Autodesk Inventor part; units mm, degrees
ref_plane "Work Plane1" through (84.9941, 63.8575, 47) normal (0, 1, 0) x (1, 0, 0)
ref_plane "Work Plane2" through (84.9941, 31.8575, 0) normal (-1, 0, 0) x (0, 0, 1)
ref_plane "YZ Plane" through (0, 0, 0) normal (1, 0, 0) x (0, 1, 0)
sketch "Sketch1" plane through (0, 0, 0) normal (0, 0, 1) x (1, 0, 0)
  line L0 (29.367, 37.7153) -> (29.0801, 37.3058)
  arc A0 (25.6709, 43.8574) -> (29.0801, 37.3058) centre (33.6709, 43.8574) ccw
  line L1 (25.6709, 51.8574) -> (25.6709, 43.8574)
  line L2 (25.6709, 43.8574) -> (25.6709, 51.8574)
  arc A1 (33.6709, 59.8574) -> (25.6709, 51.8574) centre (33.6709, 51.8574) ccw
  line L3 (33.6709, 59.8574) -> (64.6709, 59.8574)
  arc A2 (72.6709, 51.8574) -> (64.6709, 59.8574) centre (64.6709, 51.8574) ccw
  line L4 (72.6709, 43.8574) -> (72.6709, 51.8574)
  line L5 (72.6709, 51.8576) -> (72.6709, 43.8574)
  arc A3 (64.6709, 35.8574) -> (72.6709, 43.8574) centre (64.6709, 43.8574) ccw
  arc A4 (33.6709, 59.8574) -> (25.6709, 51.8574) centre (33.6709, 51.8574) ccw
  arc A5 (25.6709, 43.8574) -> (33.6709, 35.8574) centre (33.6709, 43.8574) ccw
  arc A6 (64.6709, 35.8574) -> (72.6709, 43.8574) centre (64.6709, 43.8574) ccw
  arc A7 (72.6709, 51.8574) -> (64.6709, 59.8574) centre (64.6709, 51.8574) ccw
  line L6 (33.6709, 35.8574) -> (64.6709, 35.8574)
  line L7 (33.6709, 35.8574) -> (50.3633, 35.8574)
  line L8 (50.3633, 59.8574) -> (50.3633, 35.8574)
  line L9 (25.6709, 47.8574) -> (50.3633, 47.8574)
  line L10 (84.9941, 47.8575) -> (84.9941, 63.8575)
  line L11 (84.9941, 63.8575) -> (184.9941, 63.8575)
  line L12 (84.9941, 47.8575) -> (84.9941, 31.8575)
  line L13 (84.9941, 31.8575) -> (184.9941, 31.8575)
  line L14 (184.9941, 31.8575) -> (184.9941, 63.8575)
  line L15 (184.9941, 31.8575) -> (164.9941, 31.8575)
  line L16 (164.9941, 31.8575) -> (164.9941, 21.8575)
  line L17 (164.9941, 21.8575) -> (154.9941, 21.8575)
  line L18 (154.9941, 21.8575) -> (154.9941, 31.8575)
  line L19 (84.9941, 31.8575) -> (104.9941, 31.8575)
  line L20 (104.9941, 31.8575) -> (104.9941, 21.8575)
  line L21 (104.9941, 21.8575) -> (114.9941, 21.8575)
  line L22 (114.9941, 21.8575) -> (114.9941, 31.8575)
  line L23 (184.9941, 63.8575) -> (164.9941, 63.8575)
  line L24 (164.9941, 63.8575) -> (164.9941, 73.8575)
  line L25 (164.9941, 73.8575) -> (154.9941, 73.8575)
  line L26 (154.9941, 73.8575) -> (154.9941, 63.8575)
  line L27 (84.9941, 63.8575) -> (104.9941, 63.8575)
  line L28 (104.9941, 63.8575) -> (104.9941, 73.8575)
  line L29 (104.9941, 73.8575) -> (114.9941, 73.8575)
  line L30 (114.9941, 73.8575) -> (114.9941, 63.8575)
  line L31 (104.9941, 63.8575) -> (109.9941, 63.8575)
  line L32 (104.9941, 31.8575) -> (109.9941, 31.8575)
  line L33 (104.9941, 31.8575) -> (109.9941, 31.8575)
  line L34 (109.9941, 26.8575) -> (109.9941, 31.8575)
  line L35 (154.9941, 63.8575) -> (159.9941, 63.8575)
  line L36 (154.9941, 31.8575) -> (159.9941, 31.8575)
  circle A8 centre (109.9941, 68.8575) radius 1.5875
  circle A9 centre (159.9941, 68.8575) radius 1.5875
  circle A10 centre (109.9941, 26.8575) radius 1.5875
  circle A11 centre (159.9941, 26.8575) radius 1.5875
  point P0 (0, 0)
sketch "Sketch2" plane through (0, 0, 0) normal (0, 0, 1) x (1, 0, 0)
  line L0 (29.367, 37.7153) -> (29.0801, 37.3058)
  arc A0 (25.6709, 43.8574) -> (29.0801, 37.3058) centre (33.6709, 43.8574) ccw
  line L1 (25.6709, 51.8574) -> (25.6709, 43.8574)
  line L2 (25.6709, 43.8574) -> (25.6709, 51.8574)
  arc A1 (33.6709, 59.8574) -> (25.6709, 51.8574) centre (33.6709, 51.8574) ccw
  line L3 (33.6709, 59.8574) -> (64.6709, 59.8574)
  arc A2 (72.6709, 51.8574) -> (64.6709, 59.8574) centre (64.6709, 51.8574) ccw
  line L4 (72.6709, 43.8574) -> (72.6709, 51.8574)
  line L5 (72.6709, 51.8576) -> (72.6709, 43.8574)
  arc A3 (64.6709, 35.8574) -> (72.6709, 43.8574) centre (64.6709, 43.8574) ccw
  arc A4 (33.6709, 59.8574) -> (25.6709, 51.8574) centre (33.6709, 51.8574) ccw
  arc A5 (25.6709, 43.8574) -> (33.6709, 35.8574) centre (33.6709, 43.8574) ccw
  arc A6 (64.6709, 35.8574) -> (72.6709, 43.8574) centre (64.6709, 43.8574) ccw
  arc A7 (72.6709, 51.8574) -> (64.6709, 59.8574) centre (64.6709, 51.8574) ccw
  line L6 (33.6709, 35.8574) -> (64.6709, 35.8574)
  line L7 (33.6709, 35.8574) -> (50.3633, 35.8574)
  line L8 (50.3633, 59.8574) -> (50.3633, 35.8574)
  line L9 (25.6709, 47.8574) -> (50.3633, 47.8574)
  line L10 (84.9941, 47.8575) -> (84.9941, 63.8575)
  line L11 (84.9941, 63.8575) -> (184.9941, 63.8575)
  line L12 (84.9941, 47.8575) -> (84.9941, 31.8575)
  line L13 (84.9941, 31.8575) -> (184.9941, 31.8575)
  line L14 (184.9941, 31.8575) -> (184.9941, 63.8575)
  line L15 (184.9941, 31.8575) -> (164.9941, 31.8575)
  line L16 (164.9941, 31.8575) -> (164.9941, 21.8575)
  line L17 (164.9941, 21.8575) -> (154.9941, 21.8575)
  line L18 (154.9941, 21.8575) -> (154.9941, 31.8575)
  line L19 (84.9941, 31.8575) -> (104.9941, 31.8575)
  line L20 (104.9941, 31.8575) -> (104.9941, 21.8575)
  line L21 (104.9941, 21.8575) -> (114.9941, 21.8575)
  line L22 (114.9941, 21.8575) -> (114.9941, 31.8575)
  line L23 (184.9941, 63.8575) -> (164.9941, 63.8575)
  line L24 (164.9941, 63.8575) -> (164.9941, 73.8575)
  line L25 (164.9941, 73.8575) -> (154.9941, 73.8575)
  line L26 (154.9941, 73.8575) -> (154.9941, 63.8575)
  line L27 (84.9941, 63.8575) -> (104.9941, 63.8575)
  line L28 (104.9941, 63.8575) -> (104.9941, 73.8575)
  line L29 (104.9941, 73.8575) -> (114.9941, 73.8575)
  line L30 (114.9941, 73.8575) -> (114.9941, 63.8575)
  line L31 (104.9941, 63.8575) -> (109.9941, 63.8575)
  line L32 (104.9941, 31.8575) -> (109.9941, 31.8575)
  line L33 (104.9941, 31.8575) -> (109.9941, 31.8575)
  line L34 (109.9941, 26.8575) -> (109.9941, 31.8575)
  line L35 (154.9941, 63.8575) -> (159.9941, 63.8575)
  line L36 (154.9941, 31.8575) -> (159.9941, 31.8575)
  circle A8 centre (109.9941, 68.8575) radius 1.5875
  circle A9 centre (159.9941, 68.8575) radius 1.5875
  circle A10 centre (109.9941, 26.8575) radius 1.5875
  circle A11 centre (159.9941, 26.8575) radius 1.5875
  point P0 (0, 0)
extrude "Extrusion1" add sketch "Sketch1" along normal blind 47 contours L10 L11 L14 L13 L12
extrude "Extrusion2" add sketch "Sketch2" along normal blind 5 contours L28 L29 L30 L11 | L13 L22 L21 L20 | L26 L25 L24 L11 | L13 L16 L17 L18
ref_plane "Work Plane1" through (84.9941, 63.8575, 47) normal (0, 1, 0) x (1, 0, 0)
sketch "Sketch3" plane through (84.9941, 63.8575, 47) normal (0, 1, 0) x (1, 0, 0)
  point P0 (-84.9941, 47)
ref_plane "Work Plane2" through (84.9941, 31.8575, 0) normal (-1, 0, 0) x (0, 0, 1)
sketch "Sketch4" plane through (84.9941, 31.8575, 0) normal (-1, 0, 0) x (0, 0, 1)
  line L0 (7.0327, 5.966) -> (6.7458, 5.5565)
  arc A0 (3.3366, 12.1082) -> (6.7458, 5.5565) centre (11.3366, 12.1082) ccw
  line L1 (3.3366, 20.1082) -> (3.3366, 12.1082)
  line L2 (3.3366, 12.1082) -> (3.3366, 20.1082)
  arc A1 (11.3366, 28.1082) -> (3.3366, 20.1082) centre (11.3366, 20.1082) ccw
  line L3 (11.3366, 28.1082) -> (42.3366, 28.1082)
  arc A2 (50.3366, 20.1082) -> (42.3366, 28.1082) centre (42.3366, 20.1082) ccw
  line L4 (50.3366, 12.1082) -> (50.3366, 20.1082)
  line L5 (50.3366, 20.1083) -> (50.3366, 12.1082)
  arc A3 (42.3366, 4.1082) -> (50.3366, 12.1082) centre (42.3366, 12.1082) ccw
  arc A4 (11.3366, 28.1082) -> (3.3366, 20.1082) centre (11.3366, 20.1082) ccw
  arc A5 (3.3366, 12.1082) -> (11.3366, 4.1082) centre (11.3366, 12.1082) ccw
  arc A6 (42.3366, 4.1082) -> (50.3366, 12.1082) centre (42.3366, 12.1082) ccw
  arc A7 (50.3366, 20.1082) -> (42.3366, 28.1082) centre (42.3366, 20.1082) ccw
  line L6 (11.3366, 4.1082) -> (42.3366, 4.1082)
  line L7 (11.3366, 4.1082) -> (28.029, 4.1082)
  line L8 (28.029, 28.1082) -> (28.029, 4.1082)
  line L9 (3.3366, 16.1082) -> (28.029, 16.1082)
  point P0 (0, -31.8575)
  point P1 (50.3366, 20.1082)
extrude "Extrusion3" cut sketch "Sketch4" against normal blind 110
sketch "Sketch5" plane through (84.9941, 63.8575, 47) normal (0, 1, 0) x (1, 0, 0)
  line L0 (14.3535, -16.4072) -> (87.4033, -16.4072)
  line L1 (87.4033, -16.4072) -> (87.4033, 25.9617)
  line L2 (87.4033, 25.9617) -> (14.3535, 25.9617)
  line L3 (14.3535, 25.9617) -> (14.3535, -16.4072)
  point P0 (-84.9941, 47)
extrude "Extrusion4" cut sketch "Sketch5" against normal blind 40
fillet "Fillet1" radius 2 4 edges at (92.1709, 63.8575, 47) (178.6957, 63.8575, 47) (178.6957, 31.8575, 47) (92.1709, 31.8575, 47)
fillet "Fillet2" radius 2 8 edges at (164.9941, 73.8575, 2.5) (154.9941, 73.8575, 2.5) (114.9941, 73.8575, 2.5) (104.9941, 73.8575, 2.5) (164.9941, 21.8575, 2.5) (154.9941, 21.8575, 2.5) (114.9941, 21.8575, 2.5) (104.9941, 21.8575, 2.5)
properties part number "Porta pilas"
Here's how the part is built. I have some questions about the finished solid (model axes, mm). A direction names the side the tool comes from. Give positions to 0.01 mm unless a question says otherwise; leave off trailing zeros. Write each loop counter-clockwise with the first axis right and the second up, starting at its lowest first coordinate (ties: lowest second). Pieces come first, ordered by that corner, then holes. Notation, with made-up numbers: M 45.5,89.5 L 103.5,89.5 A15 cw 103.5,98.5 Z; hole C 82,-9 d11. An arc over 180 degrees is marked long. Put each result on its own line as item: value. Start each with the question number.
Item 1: Thinking about a two-plate mould opening in Y: for faces 5 (the flat face through (160, 73.858, 2)), 6 (the cylindrical face through (134.294, 36.347, 8.897)), 7 (the flat face through (154.994, 28, 2)), which applies, +Y half, -Y half, draft (parallel to the pull), parting line (faces both ways), or undercut?
Item 2: Will these pins go through, and if not, where does the flat tip stop? pin 1 (12 mm diameter, centred on x = 143, y = 63.5, fed in from +Z); pin 2 (13.5 mm diameter, centred on x = 114, z = 27.5, fed in from -Y); pin 3 (8 mm diameter, centred on x = 112, y = 26.5, fed in from +Z); pin 4 (5 mm diameter, centred on x = 135, y = 28.5, fed in from +Z).
Item 3: If we section it at B-B, the plane x = 109.5: Write out the boundary of the cut face in (y, z).
Item 4: I need wall thicknesses on L1, parallel to Y at x = 100, z = 18.5; L2, parallel to Z at x = 145.5, y = 52; L3, parallel to Z at x = 171.5, y = 33. Which ranges of each line are inside material? Lowest first, please. Write a range as from..to.
Item 5: If we section it at A-A, the plane z = 14.5: Write out the boundary of the cut face in (x, y).
Item 6: If we section it at D-D, the plane y = 50: Write out the boundary of the cut face in (x, z).
Item 7: On a 3-axis mill with a long thin cutter (end or side, diameter ignored), from which of +Z, -Z, +X, -X, +Y, -Y can I reach the whole of each face in a straight line? I mean faces 1 (the flat face through (110, 29, 5)), 2 (the flat face through (160, 67, 5)), 3 (the flat face through (99.348, 62, 34)), 4 (the flat face through (114.994, 28, 2)). Say none if no direction works.
Item 8: If we section it at C-C, the plane z = 30.5: Write out the boundary of the cut face in (x, y).
Values:
1. face 5: +Y half
1. face 6: undercut
1. face 7: draft
2. pin 1: z = 21.04
2. pin 2: y = 31.86
2. pin 3: z = 5
2. pin 4: through
3. outline: M 21.86,0 L 25.35,0 L 25.35,5 L 21.86,5 Z; M 28.37,0 L 67.35,0 L 67.35,5 L 63.86,5 L 63.86,21.04 L 59.97,21.04 L 59.97,11.34 A8 cw 51.97,3.34 L 43.97,3.34 A8 cw 37.41,6.75 A8 cw 35.97,11.34 L 35.97,21.04 L 31.86,21.04 L 31.86,5 L 28.37,5 Z; M 70.37,0 L 73.86,0 L 73.86,5 L 70.37,5 Z
4. L1: 31.86..35.97, 59.97..63.86
4. L2: 0..3.34
4. L3: 0..21.04
5. outline: M 84.99,31.86 L 184.99,31.86 L 184.99,35.97 L 84.99,35.97 Z; M 84.99,59.97 L 184.99,59.97 L 184.99,63.86 L 84.99,63.86 Z
6. outline: M 84.99,0 L 184.99,0 L 184.99,3.34 L 84.99,3.34 Z
7. face 1: +Z, +X, -X, -Y
7. face 2: +Z, +X, -X, +Y
7. face 3: +Z, +Y, -Y
7. face 4: +Z, -Z, -Y
8. outline: M 84.99,31.86 L 99.35,31.86 L 99.35,35.97 L 84.99,35.97 Z; M 84.99,59.97 L 99.35,59.97 L 99.35,63.86 L 84.99,63.86 Z; M 172.4,31.86 L 184.99,31.86 L 184.99,35.97 L 172.4,35.97 Z; M 172.4,59.97 L 184.99,59.97 L 184.99,63.86 L 172.4,63.86 Z
